CAD build for the part. Positions are in the model's coordinates, mm. Round coordinates to 2 decimals unless told otherwise and drop trailing zeros. Order: outer loops, then holes, each group sorted by start corner. A loop starts at its lowest first (then second) coordinate and runs counter-clockwise, first axis right, second up.
```python
from build123d import *

# Parameters (mm, degrees)
RESSALTO_EXTRUS_O1_DEPTH                             = 2500
REBAIXO_PARA_PARAFUSO_DE_CABE_A_SEXTAVAD_D           = 18
REBAIXO_PARA_PARAFUSO_DE_CABE_A_SEXTAVAD_DEPTH       = 58
REBAIXO_PARA_PARAFUSO_DE_CABE_A_SEXTAVAD_CBORE_D     = 26
REBAIXO_PARA_PARAFUSO_DE_CABE_A_SEXTAVAD_CBORE_DEPTH = 25
CHANFRO1_SIZE2                                       = 2.500287455
CHANFRO1_SIZE                                        = 2.500257245
CHANFRO2_SIZE2                                       = 2.500423779
CHANFRO2_SIZE                                        = 2.500287455
CHANFRO3_SIZE                                        = 2


with BuildPart() as part:
    # Esboço1 → Ressalto-extrusão1 (new body)
    with BuildSketch(Plane.XY):
        with BuildLine():
            Line((-31.5, 20.527298986), (-31.5, 0))
            Line((-31.5, 0), (31.5, 0))
            Line((31.5, 0), (31.5, 20.527298986))
            ThreePointArc((31.5, 20.527298986), (28.900076881, 22.150342104), (27.397266061, 24.82156445))
            Line((27.397266061, 24.82156445), (24.5, 25.597882749))
            Line((24.5, 25.597882749), (24.5, 46.397686197))
            Line((24.5, 46.397686197), (27.397119712, 47.17387922))
            ThreePointArc((27.397119712, 47.17387922), (28.898613337, 49.848990738), (31.5, 51.474872705))
            Line((31.5, 51.474872705), (31.5, 58))
            Line((31.5, 58), (-31.5, 58))
            Line((-31.5, 58), (-31.5, 51.474872705))
            ThreePointArc((-31.5, 51.474872705), (-28.899411057, 49.849685923), (-27.397802135, 47.175837466))
            Line((-27.397802135, 47.175837466), (-24.5, 46.399706372))
            Line((-24.5, 46.399706372), (-24.5, 25.596973237))
            Line((-24.5, 25.596973237), (-27.397939574, 24.823365186))
            ThreePointArc((-27.397939574, 24.823365186), (-28.900095464, 22.151244343), (-31.5, 20.527298986))
        make_face()
    extrude(amount=RESSALTO_EXTRUS_O1_DEPTH)

    # Rebaixo para parafuso de cabeça sextavada de M161
    with Locations(Plane(origin=(0, 58, 0), x_dir=(1, 0, 0), z_dir=(0, 1, 0))):
        with Locations((0, -100), (0, -250), (0, -400), (0, -550), (0, -700), (0, -850), (0, -1000), (0, -1150), (0, -1300), (0, -1450), (0, -1600), (0, -1750), (0, -1900), (0, -2050), (0, -2200), (0, -2350)):
            CounterBoreHole(REBAIXO_PARA_PARAFUSO_DE_CABE_A_SEXTAVAD_D / 2, REBAIXO_PARA_PARAFUSO_DE_CABE_A_SEXTAVAD_CBORE_D / 2, REBAIXO_PARA_PARAFUSO_DE_CABE_A_SEXTAVAD_CBORE_DEPTH, depth=REBAIXO_PARA_PARAFUSO_DE_CABE_A_SEXTAVAD_DEPTH)

    # Chanfro1
    chanfro1_edges = [part.edges().sort_by_distance(p)[0] for p in [
        (-31.5, 58, 1250),
    ]]
    chamfer(chanfro1_edges, length=CHANFRO1_SIZE, length2=CHANFRO1_SIZE2)

    # Chanfro2
    chanfro2_edges = [part.edges().sort_by_distance(p)[0] for p in [
        (31.5, 58, 1250),
    ]]
    chamfer(chanfro2_edges, length=CHANFRO2_SIZE, length2=CHANFRO2_SIZE2)

    # Chanfro3
    chanfro3_edges = [part.edges().sort_by_distance(p)[0] for p in [
        (31.5, 0, 1250),
        (-31.5, 0, 1250),
    ]]
    chamfer(chanfro3_edges, length=CHANFRO3_SIZE)


solid = part.part
```
1. Cut at A-A, the plane z = 1504. Write the cut outline in (x, y), and give its area (3 significant figures).
2. Drill centre lines: line 1 (Y direction, x = 26, z = 1138); line 2 (X direction, y = 8.5, z = 1000); line 3 (X direction, y = 52.75, z = 700). Where is each one in solid material? Low to high.
3. Pin check, flat tips, straight feed: P1, Ø12, axis at x = 4.5, z = 1506.5, coming from the -Y side; P2, Ø8, axis at x = 3, z = 1902, coming from the +Y side; P3, Ø1, axis at y = 30, z = 965.5, coming from the +X side; P4, Ø23.5, axis at x = 0, z = 550, coming from the +Y side. Stop position of each tip, or through.
Outcome:
1. outline: (-31.5, 2) - (-29.5, 0) - (29.5, 0) - (31.5, 2) - (31.5, 20.53) arc R6.19 cw to (27.4, 24.82) - (24.5, 25.6) - (24.5, 46.4) - (27.4, 47.17) arc R6.19 cw to (31.5, 51.47) - (31.5, 55.5) - (29, 58) - (-29, 58) - (-31.5, 55.5) - (-31.5, 51.47) arc R6.19 cw to (-27.4, 47.18) - (-24.5, 46.4) - (-24.5, 25.6) - (-27.4, 24.82) arc R6.19 cw to (-31.5, 20.53) - close
1. area: 3,290 mm2
2. line 1: y = 0 to 25.2, 46.8 to 58
2. line 2: x = -31.5 to -9, 9 to 31.5
2. line 3: x = -31.5 to -13, 13 to 31.5
3. P1: stops at y = 0
3. P2: passes through
3. P3: stops at x = 24.5
3. P4: stops at y = 33
